Autodesk Inventor part; units mm, degrees
ref_plane "YZ Plane" through (0, 0, 0) normal (1, 0, 0) x (0, 1, 0)
ref_plane "XZ Plane" through (0, 0, 0) normal (0, 1, 0) x (-1, 0, 0)
ref_plane "XY Plane" through (0, 0, 0) normal (0, 0, 1) x (1, 0, 0)
sketch "Sketch1" plane through (0, 0, 0) normal (1, 0, 0) x (0, 1, 0)
  line L0 (-7.75, -5) -> (7.75, -5)
  line L1 (7.75, -5) -> (7.75, 5)
  line L2 (7.75, 5) -> (-7.75, 5)
  line L3 (-7.75, 5) -> (-7.75, -5)
  line L4 (-7.75, -5) -> (7.75, 5) construction
  line L5 (7.75, -5) -> (-7.75, 5) construction
  point P0 (0, 0)
  dimension "d0" = 15.5
  dimension "d1" = 10
extrude "Extrusion1" add sketch "Sketch1" along normal blind 1
sketch "Sketch2" plane through (1, 0, 0) normal (1, 0, 0) x (0, 0, -1)
  line L0 (-2.5, 2.5) -> (2.5, 2.5)
  line L1 (2.5, 2.5) -> (2.5, -2.5)
  line L2 (2.5, -2.5) -> (-2.5, -2.5)
  line L3 (-2.5, -2.5) -> (-2.5, 2.5)
  line L4 (-2.5, 2.5) -> (2.5, -2.5) construction
  line L5 (2.5, 2.5) -> (-2.5, -2.5) construction
  point P0 (0, 0)
  dimension "d4" = 5
  dimension "d5" = 5
extrude "Extrusion2" add sketch "Sketch2" along normal blind 2
sketch "Sketch3" plane through (3, 0, 0) normal (1, 0, 0) x (0, 0, -1)
  line L0 (2.5, 2.5) -> (-2.5, 2.5)
  line L1 (-2.5, 2.5) -> (-2.5, -2.5)
  line L2 (-2.5, -2.5) -> (2.5, -2.5)
  line L3 (2.5, -2.5) -> (2.5, 2.5)
  circle A0 centre (0, 0) radius 2.1413
  circle A1 centre (0, 0) radius 0.3761
extrude "Extrusion3" cut sketch "Sketch3" against normal blind 1 contours A0
sketch "Sketch4" plane through (3, 0, 2.362) normal (1, 0, 0) x (0, 1, 0)
  circle A0 centre (0, -2.362) radius 0.3761
extrude "Extrusion4" add sketch "Sketch4" along normal blind 15
ref_plane "Work Plane1" through (0, 0, 5) normal (0, 1, 0) x (1, 0, 0)
properties part number "00_LED_neopixel_single"
Input: part model. Units: mm. Frame: model coordinates. A direction names the side the tool comes from. Coordinates: 2 decimals unless noted, no trailing zeros. Loops run counter-clockwise (first coordinate to the right, second up) from the corner with the lowest first, then second, coordinate; pieces in that order, holes last. Notation, with made-up numbers: (84.5, 10) - (124.5, 10) arc R15 cw to (124.5, 28) - close; hole circle Ø8 at (73, 44). An arc over 180 degrees is marked (long way). Answer in a Markdown table with one row per item.
(1) Cut plane A-A on x = 2.5. Output: boundary loops of the cut face in (y, z), plus the area to 3 significant figures.
Model answer:
| item | result |
|---|---|
| outline | (-2.5, -2.5) - (2.5, -2.5) - (2.5, 2.5) - (-2.5, 2.5) - close; circle Ø0.75 at (0, 0); hole circle Ø4.28 at (0, 0) |
| area | 11.0 mm² |
(2) Material intervals for L1, parallel to Y at x = 2.6, z = 0; L2, parallel to X at y = -4.75, z = -2.5; L3, parallel to Y at x = 2.75, z = -2.25, sorted ascending. Write a range as from..to.
Model answer:
| item | result |
|---|---|
| L1 | y = -2.5..-2.14, -0.38..0.38, 2.14..2.5 |
| L2 | x = 0..1 |
| L3 | y = -2.5..2.5 |
(3) Set-up query: faces 1 (the face through (2, 0, 2.5)), 2 (the face through (0, 0, 0)), 3 (the face through (2, -2.5, 0)), 4 (the face through (2, 1, 0)). Return all of +Z, -Z, +X, -X, +Y, -Y with unobstructed straight access to the full face (end or side cutting, diameter ignored); none if empty.
Model answer:
| item | result |
|---|---|
| face 1 | +Z, +X, +Y, -Y |
| face 2 | +Z, -Z, -X, +Y, -Y |
| face 3 | +Z, -Z, +X, -Y |
| face 4 | +X |
(4) Pin query (flat end, axial travel): P1, Ø0.6, axis at x = 1.5, z = 0.5, coming from the +Y side; P2, Ø0.6, axis at x = 1.5, z = 1, coming from the -Y side; P3, Ø5, axis at y = -3, z = -1, coming from the +X side. Return the tip coordinate at first contact, or that it passes through.
Model answer:
| item | result |
|---|---|
| P1 | stops at y = 2.5 |
| P2 | stops at y = -2.5 |
| P3 | stops at x = 3 |
(5) Mould query, pull axis Y, two halves, no side actions, for faces 5 (the face through (2.5, -1.3, 1.7)), 6 (the face through (2, 2.5, 0)), 7 (the face through (2, 0, -2.5)). Classes: pulls with the +Y half, pulls with the -Y half, needs draft (parallel to the pull), parting line crosses it, or undercut.
Model answer:
| item | result |
|---|---|
| face 5 | undercut |
| face 6 | pulls with the +Y half |
| face 7 | needs draft |
(6) Cut plane B-B on y = 0. Output: boundary loops of the cut face in (x, z), plus the area to 3 significant figures.
Model answer:
| item | result |
|---|---|
| outline | (0, -5) - (1, -5) - (1, -2.5) - (3, -2.5) - (3, -2.14) - (2, -2.14) - (2, -0.38) - (18, -0.38) - (18, 0.38) - (2, 0.38) - (2, 2.14) - (3, 2.14) - (3, 2.5) - (1, 2.5) - (1, 5) - (0, 5) - close |
| area | 27.8 mm² |
(7) Cut plane D-D on x = 14.25. Output: boundary loops of the cut face in (y, z).
Model answer:
| item | result |
|---|---|
| outline | circle Ø0.75 at (0, 0) |
(8) Cut plane C-C on z = 0. Output: boundary loops of the cut face in (x, y), plus the area to 3 significant figures.
Model answer:
| item | result |
|---|---|
| outline | (0, -7.75) - (1, -7.75) - (1, -2.5) - (3, -2.5) - (3, -2.14) - (2, -2.14) - (2, -0.38) - (18, -0.38) - (18, 0.38) - (2, 0.38) - (2, 2.14) - (3, 2.14) - (3, 2.5) - (1, 2.5) - (1, 7.75) - (0, 7.75) - close |
| area | 33.3 mm² |
